```python
from build123d import *

# Parameters (mm, degrees)
SKETCH1_W             = 11.89875271
SKETCH1_H             = 10
SKETCH1_R             = 1.375
BOSS_EXTRUDE1_DEPTH   = 3
SKETCH1_W_2           = 11.9
BOSS_EXTRUDE1_2_DEPTH = 3
SKETCH1_4_W           = 3.00124729
SKETCH1_4_H           = 10
SKETCH1_4_W_2         = 3
BOSS_EXTRUDE2_DEPTH   = 18.7
BOSS_EXTRUDE3_REACH   = 42.581
SKETCH3_W             = 10
SKETCH3_H             = 3


with BuildPart() as part:
    # Sketch1 → Boss-Extrude1 (new body)
    with BuildSketch(Plane(origin=(0, 0, 0), x_dir=(1, 0, 0), z_dir=(0, 1, 0))):
        with Locations((5.949376355, -5)):
            Rectangle(SKETCH1_W, SKETCH1_H)
        with Locations(Location((6.75, -5, 0), (0, 0, 270))):
            Circle(SKETCH1_R, mode=Mode.SUBTRACT)
    extrude(amount=BOSS_EXTRUDE1_DEPTH)



with BuildPart() as body_2:
    # Sketch1 → Boss-Extrude1 2 (new body)
    with BuildSketch(Plane(origin=(0, 0, 0), x_dir=(1, 0, 0), z_dir=(0, 1, 0))):
        with Locations((43.55, -5)):
            Rectangle(SKETCH1_W_2, SKETCH1_H)
        with Locations(Location((42.75, -5, 0), (0, 0, 270))):
            Circle(SKETCH1_R, mode=Mode.SUBTRACT)
    extrude(amount=BOSS_EXTRUDE1_2_DEPTH)


with BuildPart() as part_1:
    add(part.part)

    add(body_2.part)  # Boss-Extrude2 merges body 2
    # Sketch1_4 → Boss-Extrude2 (add)
    with BuildSketch(Plane(origin=(0, 0, 0), x_dir=(1, 0, 0), z_dir=(0, 1, 0))):
        with Locations((13.399376355, -5)):
            Rectangle(SKETCH1_4_W, SKETCH1_4_H)
        with Locations((36.1, -5)):
            Rectangle(SKETCH1_4_W_2, SKETCH1_4_H)
    extrude(amount=BOSS_EXTRUDE2_DEPTH)

    # Sketch3 → Boss-Extrude3 (add, up to next)
    with BuildSketch(Plane(origin=(14.9, 0, 0), x_dir=(0, 0, -1), z_dir=(1, 0, 0)), mode=Mode.PRIVATE) as boss_extrude3_sk1:
        with Locations((-5, 17.2)):
            Rectangle(SKETCH3_W, SKETCH3_H)
    boss_extrude3_tool1 = extrude(boss_extrude3_sk1.sketch, amount=BOSS_EXTRUDE3_REACH, mode=Mode.PRIVATE) - part_1.part
    add(boss_extrude3_tool1.solids().sort_by_distance((14.9, 17.2, 5))[0])


solid = part_1.part
```
The listing builds one solid part. Answer for the finished solid, in the listing's coordinates (mm). A direction names the side the tool comes from. Coordinates: 2 decimals unless noted, no trailing zeros. Loops run counter-clockwise (first coordinate to the right, second up) from the corner with the lowest first, then second, coordinate; pieces in that order, holes last. Notation, with made-up numbers: M -4.5,-18 L 39.5,-18 A17 cw 39.5,-6 Z; hole C 8,-38.5 d10. An arc over 180 degrees is marked long. Answer as a JSON object with one key per item and string values. Group by question number.
Item 1: Section C-C (x = 6.75) is taken. Write down the section's boundary in (y, z) (3 decimals).
Item 2: Determine the mould class of faces 4 (the face through (49.5, 1, 5)), 5 (the face through (0, 1, 5)), 6 (the face through (8.113, 1.479, 4.821)) for opening direction X: +X half, -X half, draft (parallel to the pull), parting line (faces both ways), or undercut.
Item 3: Each of these flat-tipped pins is pushed along its axis until it touches: P1, Ø2, axis at y = 10, z = 8, coming from the +X side; P2, Ø5, axis at x = 27, z = 4, coming from the -Y side; P3, Ø8, axis at x = 22, y = 3.5, coming from the +Z side; P4, Ø5, axis at x = 43, z = 4, coming from the +Y side. Where does it stop, or does it pass through?
Item 4: Consider L1, parallel to X at y = 2.35, z = 5 (3 decimals); L2, parallel to X at y = 12.25, z = 5.25; L3, parallel to X at y = 2.75, z = 7. Determine where each line is inside the solid, lowest interval first.
Item 5: Section B-B (z = 5) is taken. Write down the section's boundary in (x, y) (3 decimals).
Item 6: Section D-D (y = 4.75) is taken. Write down the section's boundary in (x, z).
Item 7: Section A-A (y = 2.5) is taken. Write down the section's boundary in (x, z) (3 decimals).
Item 8: Which of the six approach directions +Z, -Z, +X, -X, +Y, -Y give full straight-line access (tool end or side, diameter ignored) to faces 1 (the face through (5, 3, 5)), 2 (the face through (25, 15.7, 5)), 3 (the face through (45, 3, 5))?
Solved:
{
 "1": {"outline": "M 0,0 L 3,0 L 3,3.625 L 0,3.625 Z; M 0,6.375 L 3,6.375 L 3,10 L 0,10 Z"},
 "2": {"face 4": "+X half", "face 5": "-X half", "face 6": "undercut"},
 "3": {"P1": "stops at x = 37.6", "P2": "stops at y = 15.7", "P3": "passes through", "P4": "stops at y = 3"},
 "4": {"L1": "x = 0 to 5.375, 8.125 to 14.9, 34.6 to 41.375, 44.125 to 49.5", "L2": "x = 11.9 to 14.9, 34.6 to 37.6", "L3": "x = 0 to 14.9, 34.6 to 49.5"},
 "5": {"outline": "M 0,0 L 5.375,0 L 5.375,3 L 0,3 Z; M 8.125,0 L 14.9,0 L 14.9,15.7 L 34.6,15.7 L 34.6,0 L 41.375,0 L 41.375,3 L 37.6,3 L 37.6,18.7 L 11.899,18.7 L 11.899,3 L 8.125,3 Z; M 44.125,0 L 49.5,0 L 49.5,3 L 44.125,3 Z"},
 "6": {"outline": "M 11.9,0 L 14.9,0 L 14.9,10 L 11.9,10 Z; M 34.6,0 L 37.6,0 L 37.6,10 L 34.6,10 Z"},
 "7": {"outline": "M 0,0 L 14.9,0 L 14.9,10 L 0,10 Z; M 34.6,0 L 49.5,0 L 49.5,10 L 34.6,10 Z; hole C 6.75,5 d2.75; hole C 42.75,5 d2.75"},
 "8": {"face 1": "+Z, -Z, -X, +Y", "face 2": "+Z, -Z, -Y", "face 3": "+Z, -Z, +X, +Y"}
}
